Autodesk Inventor part; units mm, degrees
ref_plane "YZ Plane" through (0, 0, 0) normal (1, 0, 0) x (0, 1, 0)
ref_plane "XZ Plane" through (0, 0, 0) normal (0, 1, 0) x (-1, 0, 0)
ref_plane "XY Plane" through (0, 0, 0) normal (0, 0, 1) x (1, 0, 0)
sketch "Sketch1" plane through (0, 0, 0) normal (0, 1, 0) x (-1, 0, 0)
  line L0 (8.89, 21.59) -> (-8.89, 21.59)
  line L1 (-8.89, 21.59) -> (-8.89, -21.59)
  line L2 (-8.89, -21.59) -> (8.89, -21.59)
  line L3 (8.89, -21.59) -> (8.89, 21.59)
  circle A0 centre (7.62, 20.32) radius 0.889
  circle A1 centre (-7.62, 20.32) radius 0.889
  line L4 (8.89, 0) -> (-8.89, 0) construction
  circle A2 centre (7.62, -20.32) radius 0.889
  circle A3 centre (-7.62, -20.32) radius 0.889
  point P0 (0, 0)
  dimension "d0" = 17.78
  dimension "d1" = 43.18
  dimension "d2" = 21.59
  dimension "d3" = 8.89
  dimension "d4" = 15.24
  dimension "d5" = 7.62
  dimension "d6" = 1.778
  dimension "d7" = 1.778
  dimension "d8" = 1.27
  dimension "d9" = 1.27
  dimension "d10" = 1.27
  dimension "d11" = 40.64
  dimension "d12" = 13.462
  dimension "d15" = 15.24
extrude "Extrusion1" add sketch "Sketch1" along normal blind 3
equation "\"d9\" = d8"
properties part number "arduino nano screw ports"
Input: part model. Units: mm. Frame: model coordinates. Coordinates: 2 decimals unless noted, no trailing zeros. Write each loop counter-clockwise with the first axis right and the second up, starting at its lowest first coordinate (ties: lowest second). Pieces come first, ordered by that corner, then holes.
1) Section A-A on x = -7.62. Output: boundary loops of the cut face in (y, z).
2) Material intervals for line 1 along Z through (x, y) = (-7.62, 0.8); line 2 along Z through (x, y) = (-7.25, 1.6); line 3 along X through (y, z) = (2.7, -20), sorted ascending.
3) Section B-B on z = 20.32. Output: boundary loops of the cut face in (x, y), and give its area (3 significant figures).
4) Mould query, pull axis X, two halves, no side actions, for faces 1 (the flat face through (-8.89, 1, 0)), 2 (the flat face through (0, 1, -21.59)), 3 (the cylindrical face through (8.325, 1.479, 20.861)). Classes: pulls with the +X half, pulls with the -X half, needs draft (parallel to the pull), parting line crosses it, or undercut.
5) Pin query (flat end, axial travel): pin 1 Ø1.4 at (x, z) = (7.62, 20.32) entering from -Y. Return the tip coordinate at first contact, or that it passes through.
Check result:
1. outline: (0, -21.59) - (3, -21.59) - (3, -21.21) - (0, -21.21) - close; (0, -19.43) - (3, -19.43) - (3, 19.43) - (0, 19.43) - close; (0, 21.21) - (3, 21.21) - (3, 21.59) - (0, 21.59) - close
2. line 1: z = -21.59 to -21.21, -19.43 to 19.43, 21.21 to 21.59
2. line 2: z = -21.59 to -21.13, -19.51 to 19.51, 21.13 to 21.59
2. line 3: x = -8.89 to -8.45, -6.79 to 6.79, 8.45 to 8.89
3. outline: (-8.89, 0) - (-8.51, 0) - (-8.51, 3) - (-8.89, 3) - close; (-6.73, 0) - (6.73, 0) - (6.73, 3) - (-6.73, 3) - close; (8.51, 0) - (8.89, 0) - (8.89, 3) - (8.51, 3) - close
3. area: 42.7 mm2
4. face 1: pulls with the -X half
4. face 2: needs draft
4. face 3: undercut
5. pin 1: passes through
